Autodesk Inventor part; units mm, degrees
ref_plane "FDT_PIRODACC_M1_XY" through (-15, 0, 0) normal (-1, 0, 0) x (0, 1, 0)
ref_plane "FDT_PIRODACC_M1_YZ" through (-15, 0, 0) normal (0, 1, 0) x (0, 0, -1)
ref_plane "FDT_PIRODACC_M1_ZX" through (-15, 0, 0) normal (0, 0, -1) x (-1, 0, 0)
sketch "Sketch_1" plane through (0, 0, 0) normal (0, 0, 1) x (1, 0, 0)
  line L0 (42.6, 0) -> (-6, 0)
  line L1 (-6, 0) -> (-6, 6)
  line L2 (-6, 6) -> (42.6, 6)
  line L3 (42.6, 6) -> (42.6, 0)
  line L4 (42.6, 0) -> (-6, 0)
revolve "Revolution1" add sketch "Sketch_1" angle 360 about axis through (42.6, 0, 0) along (1, 0, 0)
sketch "Sketch_11" plane through (0, 0, 0) normal (0, 0, 1) x (1, 0, 0)
  line L0 (42.6, 0) -> (34.6, 0)
  line L1 (34.6, 0) -> (34.6, 16)
  line L2 (34.6, 16) -> (42.6, 16)
  line L3 (42.6, 16) -> (42.6, 0)
  line L4 (42.6, 0) -> (34.6, 0)
revolve "Revolution2" add sketch "Sketch_11" angle 360 about axis through (42.6, 0, 0) along (1, 0, 0)
sketch "Sketch_19" plane through (0, 0, 0) normal (0, 0, 1) x (1, 0, 0)
  line L0 (-5, 0) -> (-25, 0)
  line L1 (-25, 0) -> (-25, 4.233)
  line L2 (-25, 4.233) -> (-24.233, 5)
  line L3 (-24.233, 5) -> (-9.9727, 5)
  line L4 (-9.9727, 5) -> (-7.5994, 4.1362)
  arc A0 (-7.5994, 4.1362) -> (-7.3942, 4.1) centre (-7.3942, 4.7) ccw
  line L5 (-7.3942, 4.1) -> (-6.6, 4.1)
  arc A1 (-6.6, 4.1) -> (-6, 4.7) centre (-6.6, 4.7) ccw
  line L6 (-6, 4.7) -> (-6, 5)
  line L7 (-6, 5) -> (-5, 5)
  line L8 (-5, 5) -> (-5, 0)
  line L9 (-5, 0) -> (-25, 0)
revolve "Revolution3" add sketch "Sketch_19" angle 360 about axis through (-5, 0, 0) along (1, 0, 0)
thread "Thread1"
sketch "Sketch_20" plane through (0, 0, 0) normal (0, 0, 1) x (1, 0, 0)
  line L0 (-36, -16) -> (5.0509, -16)
  line L1 (5.0509, -16) -> (-1.3, -5)
  line L2 (-1.3, -5) -> (-6, -5)
  line L3 (-6, -5) -> (-6, -10)
  line L4 (-6, -10) -> (-30, -10)
  line L5 (-30, -10) -> (-30, 10)
  line L6 (-30, 10) -> (-6, 10)
  line L7 (-6, 10) -> (-6, 5)
  line L8 (-6, 5) -> (-1.3, 5)
  line L9 (-1.3, 5) -> (5.0509, 16)
  line L10 (5.0509, 16) -> (-36, 16)
  line L11 (-36, 16) -> (-36, -16)
extrude "Extrusion1" cut sketch "Sketch_20" along normal mid plane 24
ref_plane "FDT_PIRODACC_M1_XY" through (-15, 0, 0) normal (-1, 0, 0) x (0, 1, 0)
ref_plane "FDT_PIRODACC_M1_YZ" through (-15, 0, 0) normal (0, 1, 0) x (0, 0, -1)
ref_plane "FDT_PIRODACC_M1_ZX" through (-15, 0, 0) normal (0, 0, -1) x (-1, 0, 0)
ref_plane "NUT1_XY" through (-12.5, 0, 0) normal (1, 0, 0) x (0, 0, -1)
ref_plane "NUT1_YZ" through (-12.5, 0, 0) normal (0, 0, -1) x (0, 1, 0)
ref_plane "NUT1_ZX" through (-12.5, 0, 0) normal (0, 1, 0) x (1, 0, 0)
ref_plane "PISTON_XY" through (42.6, 0, 0) normal (1, 0, 0) x (0, 0, -1)
ref_plane "PISTON_YZ" through (42.6, 0, 0) normal (0, 0, -1) x (0, 1, 0)
ref_plane "PISTON_ZX" through (42.6, 0, 0) normal (0, 1, 0) x (1, 0, 0)
properties part number "536267 ADN-15-P-A_(KS)"
Work out the finished part from the listing and answer in its coordinate system (mm). A direction names the side the tool comes from. Coordinates: 2 decimals unless noted, no trailing zeros. Order: outer loops, then holes, each group sorted by start corner. A loop starts at its lowest first (then second) coordinate and runs counter-clockwise, first axis right, second up. Notation, with made-up numbers: M 46.5,38.5 L 91.5,38.5 A24 ccw 91.5,58.5 Z; hole C 13.5,75 d5. An arc over 180 degrees is marked long. Use CSV: the item, a comma, the result in double quotes.
1) Section C-C on x = -14.5 is taken. Write down the section's boundary in (y, z).
Worked out:
outline,"C 0,0 d10"
2) Determine the mould class of faces 1 (the face through (42.6, 0, 0)), 2 (the face through (-7.748, -0.545, -4.155)), 3 (the face through (-4, -5, 0)) for opening direction X: released by +X, released by -X, zero draft, split by the parting line, or undercut.
Worked out:
face 1,"released by +X"
face 2,"undercut"
face 3,"zero draft"
3) For faces 4 (the face through (15, -6, 0)), 5 (the face through (-25, 0, 0)), 6 (the face through (-6, 0, -5)), 7 (the face through (-4, 5, 0)), determine the directions among +Z, -Z, +X, -X, +Y, -Y from which every point of the face is accessible in a straight line to the end or side of a thin tool.
Worked out:
face 4,"-X"
face 5,"+Z, -Z, -X, +Y, -Y"
face 6,"none"
face 7,"+Z, -Z, -X, +Y"
4) Consider line 1 (X direction, y = 5, z = 13); line 2 (X direction, y = -3.5, z = -4.5); line 3 (Z direction, x = -11, y = -2.5). Determine where each line is inside the solid, lowest interval first. Write a range as [from, to].
Worked out:
line 1,"x = [34.6, 42.6]"
line 2,"x = [-6, 42.6]"
line 3,"z = [-4.33, 4.33]"
5) Flat-ended cylindrical pins translate along their axes: pin 1 Ø6 at (x, z) = (30, 8) entering from -Y; pin 2 Ø10 at (x, y) = (-7.5, 8) entering from +Z; pin 3 Ø1 at (x, y) = (1, -2.5) entering from +Z. Find the tip coordinate at first contact, or state that the pin passes through.
Worked out:
pin 1,"stops at y = -3.32"
pin 2,"stops at z = 5.06"
pin 3,"stops at z = 5.66"
6) Section D-D on x = 4.5 is taken. Write down the section's boundary in (y, z).
Worked out:
outline,"C 0,0 d12"
7) Section A-A on z = 0 is taken. Write down the section's boundary in (x, y).
Worked out:
outline,"M -25,-4.23 L -24.23,-5 L -9.97,-5 L -7.6,-4.14 A0.6 cw -7.39,-4.1 L -6.6,-4.1 A0.6 cw -6,-4.7 L -6,-5 L -1.3,-5 L -0.72,-6 L 34.6,-6 L 34.6,-16 L 42.6,-16 L 42.6,16 L 34.6,16 L 34.6,6 L -0.72,6 L -1.3,5 L -6,5 L -6,4.7 A0.6 cw -6.6,4.1 L -7.39,4.1 A0.6 cw -7.6,4.14 L -9.97,5 L -24.23,5 L -25,4.23 Z"
8) Section B-B on y = 0 is taken. Write down the section's boundary in (x, z).
Worked out:
outline,"M -25,-4.23 L -24.23,-5 L -9.97,-5 L -7.6,-4.14 A0.6 cw -7.39,-4.1 L -6.6,-4.1 A0.6 cw -6,-4.7 L -6,-6 L 34.6,-6 L 34.6,-16 L 42.6,-16 L 42.6,16 L 34.6,16 L 34.6,6 L -6,6 L -6,4.7 A0.6 cw -6.6,4.1 L -7.39,4.1 A0.6 cw -7.6,4.14 L -9.97,5 L -24.23,5 L -25,4.23 Z"
